```python
from build123d import *

# Parameters (mm, degrees)
F4_R     = 3
F4_R_2   = 1
F5_DEPTH = 1.7
F6_DEPTH = 0.5
F8_DEPTH = 62
F4_R_3   = 0.75
F9_DEPTH = 1.4
F10_R    = 0.25


with BuildPart() as f5:
    # F4 (on Top) → F5 (new body)
    with BuildSketch(Plane.XY):
        with BuildLine():
            ThreePointArc((-43.2966782842, 88.958070665), (-46.4043790169, 87.9618261956), (-47.7356673777, 84.9822325677))
            Line((-47.7356673777, 84.9822325677), (-47.7356673777, -13.3634495586))
            ThreePointArc((-47.7356673777, -13.3634495586), (-45.7684587141, -18.9794842824), (-40.7268127068, -22.1404274143))
            Line((-40.7268127068, -22.1404274143), (-13.8418592272, -28.2395483673))
            ThreePointArc((-13.8418592272, -28.2395483673), (-12.7356673777, -28.3634495586), (-11.6294755282, -28.2395483673))
            Line((-11.6294755282, -28.2395483673), (15.2554779514, -22.1404274143))
            ThreePointArc((15.2554779514, -22.1404274143), (20.2971239587, -18.9794842824), (22.2643326223, -13.3634495586))
            Line((22.2643326223, -13.3634495586), (22.2643326223, 78.1365504414))
            ThreePointArc((22.2643326223, 78.1365504414), (21.2439262501, 80.8052620805), (18.7033217158, 82.1123885387))
            Line((18.7033217158, 82.1123885387), (-43.2966782842, 88.958070665))
        make_face()
        with Locations((-12.7356673777, -23.3634495586)):
            Circle(F4_R, mode=Mode.SUBTRACT)
        with BuildLine():
            Line((-43.7356673777, 73.1365504414), (-43.7356673777, 78.1365504414))
            Line((-43.7356673777, 78.1365504414), (18.2643326223, 78.1365504414))
            Line((18.2643326223, 78.1365504414), (18.2643326223, 73.1365504414))
            Line((18.2643326223, 73.1365504414), (18.2643326223, -13.3634495586))
            ThreePointArc((18.2643326223, -13.3634495586), (16.7998665282, -16.8989834645), (13.2643326223, -18.3634495586))
            Line((13.2643326223, -18.3634495586), (-38.7356673777, -18.3634495586))
            ThreePointArc((-38.7356673777, -18.3634495586), (-42.2712012836, -16.8989834645), (-43.7356673777, -13.3634495586))
            Line((-43.7356673777, -13.3634495586), (-43.7356673777, 73.1365504414))
        make_face(mode=Mode.SUBTRACT)
        with Locations((-42.6353360717, 81.1365504414)):
            Circle(F4_R_2, mode=Mode.SUBTRACT)
        with Locations((-43.7356673777, 84.9822325677)):
            Circle(F4_R_2, mode=Mode.SUBTRACT)
    extrude(amount=F5_DEPTH)

    # F4 (on Top) → F6 (join)
    with BuildSketch(Plane.XY):
        with BuildLine():
            Line((18.2643326223, 73.1365504414), (-43.7356673777, 73.1365504414))
            Line((-43.7356673777, 73.1365504414), (-43.7356673777, -13.3634495586))
            ThreePointArc((-43.7356673777, -13.3634495586), (-42.2712012836, -16.8989834645), (-38.7356673777, -18.3634495586))
            Line((-38.7356673777, -18.3634495586), (13.2643326223, -18.3634495586))
            ThreePointArc((13.2643326223, -18.3634495586), (16.7998665282, -16.8989834645), (18.2643326223, -13.3634495586))
            Line((18.2643326223, -13.3634495586), (18.2643326223, 73.1365504414))
        make_face()
    extrude(amount=F6_DEPTH)

    # F7 (on face) → F8 (join, through all)
    with BuildSketch(Plane(origin=(18.2643326223, 0, 0), x_dir=(0, -1, 0), z_dir=(-1, 0, 0))):
        Polygon((-73.1365504414, 0), (-73.1365504414, 0.5), (-78.1365504414, 1.7), (-78.1365504414, 0), align=None)
    extrude(amount=F8_DEPTH)

    # F4 (on Top) → F9 (join, through all)
    with BuildSketch(Plane.XY):
        with Locations((-43.7356673777, 84.9822325677)):
            Circle(F4_R_2)
        with Locations((-43.7356673777, 84.9822325677)):
            Circle(F4_R_3, mode=Mode.SUBTRACT)
        with Locations((-42.6353360717, 81.1365504414)):
            Circle(F4_R_2)
        with Locations((-42.6353360717, 81.1365504414)):
            Circle(F4_R_3, mode=Mode.SUBTRACT)
    extrude(amount=F9_DEPTH)

    # F10
    f10_edges = [f5.edges().sort_by_distance(p)[0] for p in [
        (-43.735667, 32.38655, 1.7),
        (22.264333, 32.38655, 1.7),
        (-27.284336, -25.189988, 0),
    ]]
    fillet(f10_edges, radius=F10_R)


solid = f5.part
```
Input: part model. Units: mm. Frame: model coordinates. A direction names the side the tool comes from. Give positions to 0.01 mm unless a question says otherwise; leave off trailing zeros. Order: outer loops, then holes, each group sorted by start corner. A loop starts at its lowest first (then second) coordinate and runs counter-clockwise, first axis right, second up.
1. Line query: probe 1 along X at (y, z) = (35.5, 1.5); probe 2 along X at (y, z) = (73, 1.55); probe 3 along Z at (x, y) = (-3.5, -6.5). Output: solid intervals per line, ascending.
Computed:
probe 1: x = -47.73 to -43.74, 18.27 to 22.26
probe 2: x = -47.71 to -43.76, 18.29 to 22.24
probe 3: z = 0 to 0.5
2. Set-up query: faces 4 (the face through (-42.23, -16.94, 0.97)), 5 (the face through (20.24, -19.05, 0.84)). Return all of +Z, -Z, +X, -X, +Y, -Y with unobstructed straight access to the full face (end or side cutting, diameter ignored); none if empty.
Computed:
face 4: +Z
face 5: +Z, -Z, +X, -Y
3. Cut plane B-B (z = 1.05). Return loops of the section in (x, y).
Computed:
outline: (-47.74, -13.36) arc R9 ccw to (-40.73, -22.14) - (-13.84, -28.24) arc R5 ccw to (-11.63, -28.24) - (15.26, -22.14) arc R9 ccw to (22.26, -13.36) - (22.26, 78.14) arc R4 ccw to (18.7, 82.11) - (-43.3, 88.96) arc R4 ccw to (-47.74, 84.98) - close; hole circle Ø1.5 at (-43.74, 84.98); hole (-43.74, -13.36) arc R5 ccw to (-38.74, -18.36) - (13.26, -18.36) arc R5 ccw to (18.26, -13.36) - (18.26, 75.43) - (-43.74, 75.43) - close; hole circle Ø1.5 at (-42.64, 81.14); hole circle Ø6 at (-12.74, -23.36)
4. Pin query (flat end, axial travel): pin 1 Ø3.5 at (x, y) = (-12.74, -23.36) entering from -Z; pin 2 Ø3 at (x, y) = (-38, 31.5) entering from +Z; pin 3 Ø0.8 at (x, z) = (-7.5, 1) entering from +Y. Return the tip coordinate at first contact, or that it passes through.
Computed:
pin 1: passes through
pin 2: stops at z = 0.5
pin 3: stops at y = 85.05
5. Cut plane A-A (y = -9.5). Return loops of the section in (x, z), and give its area (3 significant figures).
Computed:
outline: (-47.74, 0.25) arc R0.25 ccw to (-47.49, 0) - (22.01, 0) arc R0.25 ccw to (22.26, 0.25) - (22.26, 1.45) arc R0.25 ccw to (22.01, 1.7) - (18.51, 1.7) arc R0.25 ccw to (18.26, 1.45) - (18.26, 0.5) - (-43.74, 0.5) - (-43.74, 1.45) arc R0.25 ccw to (-43.99, 1.7) - (-47.49, 1.7) arc R0.25 ccw to (-47.74, 1.45) - close
area: 44.5 mm2
6. Draft query along X for faces 1 (the face through (-11.863, 85.487, 0.842)), 2 (the face through (-13, 28, 0.5)), 3 (the face through (-13, 31, 0)). Return one class per face: released by +X, released by -X, zero draft, split by the parting line, or undercut.
Computed:
face 1: released by +X
face 2: undercut
face 3: zero draft
